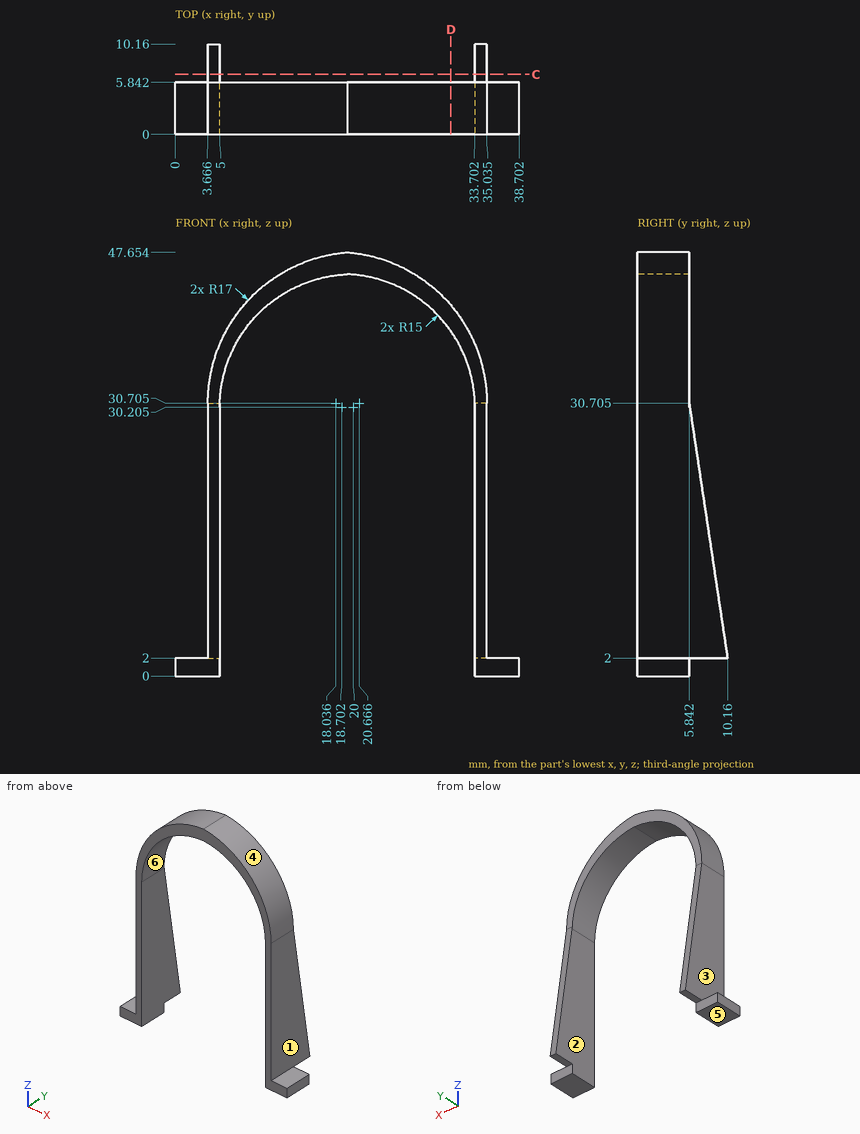
Geometry: see drawing. Coordinates: mm, zero at the bounding-box minimum. A direction names the side the tool comes from. Give positions to 0.01 mm unless a question says otherwise; leave off trailing zeros. Order: outer loops, then holes, each group sorted by start corner. A loop starts at its lowest first (then second) coordinate and runs counter-clockwise, first axis right, second up. Notation, with made-up numbers: (74, 80) - (85, 80) arc R15 ccw to (85, 93) - close; hole circle Ø8 at (-17.5, 71). An arc over 180 degrees is marked (long way). One line per item, written item: value.
1. Cut plane C-C, the plane y = 6.75. Output: boundary loops of the cut face in (x, z) (1 decimal).
Determined:
outline: (3.7, 2) - (5, 2) - (5, 24.7) - (3.7, 24.7) - close; (33.7, 2) - (35, 2) - (35, 24.7) - (33.7, 24.7) - close
2. Draft query along X for the marked faces 4, 5 and 6. Return one class per face: released by +X, released by -X, zero draft, split by the parting line, or undercut.
Determined:
face 4: released by +X
face 5: zero draft
face 6: undercut
3. Pin query (flat end, axial travel): pin 1 Ø3 at (x, y) = (5, 8.5) entering from -Z; pin 2 Ø3 at (x, y) = (26, 9) entering from -Z; pin 3 Ø3 at (x, y) = (37.5, 4) entering from +Z; pin 4 Ø19 at (x, z) = (24, 39.5) entering from +Y. Return the tip coordinate at first contact, or that it passes through.
Determined:
pin 1: z = 2
pin 2: through
pin 3: z = 2
pin 4: y = 5.84
4. Reachability of the marked faces 1, 2 and 3 from +Z, -Z, +X, -X, +Y, -Y: full face, straight path, thin tool, end or side. Return the list, or none.
Determined:
face 1: +Z, +X, +Y, -Y
face 2: -Z, +Y, -Y
face 3: +Z, -X, +Y, -Y
5. Line query: probe 1 along X at (y, z) = (1.75, 19.5) (1 decimal); probe 2 along Z at (x, y) = (2, 5.75); probe 3 along Z at (x, y) = (11, 2.5) (1 decimal). Output: solid intervals per line, ascending.
Determined:
probe 1: 3.7 to 5, 33.7 to 35
probe 2: 0 to 2
probe 3: 42.2 to 44.7
6. Cut plane D-D, the plane x = 31. Output: boundary loops of the cut face in (y, z).
Determined:
outline: (0, 38.79) - (5.84, 38.79) - (5.84, 41.7) - (0, 41.7) - close
